Verification items for this drawing (mm, ordinates from the low corner). Round coordinates to 2 decimals unless told otherwise and drop trailing zeros. Write each loop counter-clockwise with the first axis right and the second up, starting at its lowest first coordinate (ties: lowest second). Pieces come first, ordered by that corner, then holes. Notation, with made-up numbers: (-11.5, 66.25) -> (25.5, 66.25) arc R11 ccw to (25.5, 70.25) -> close; hole circle Ø1 at (3, 48.5). An arc over 180 degrees is marked (long way). One line per question, with ' | ' between items.
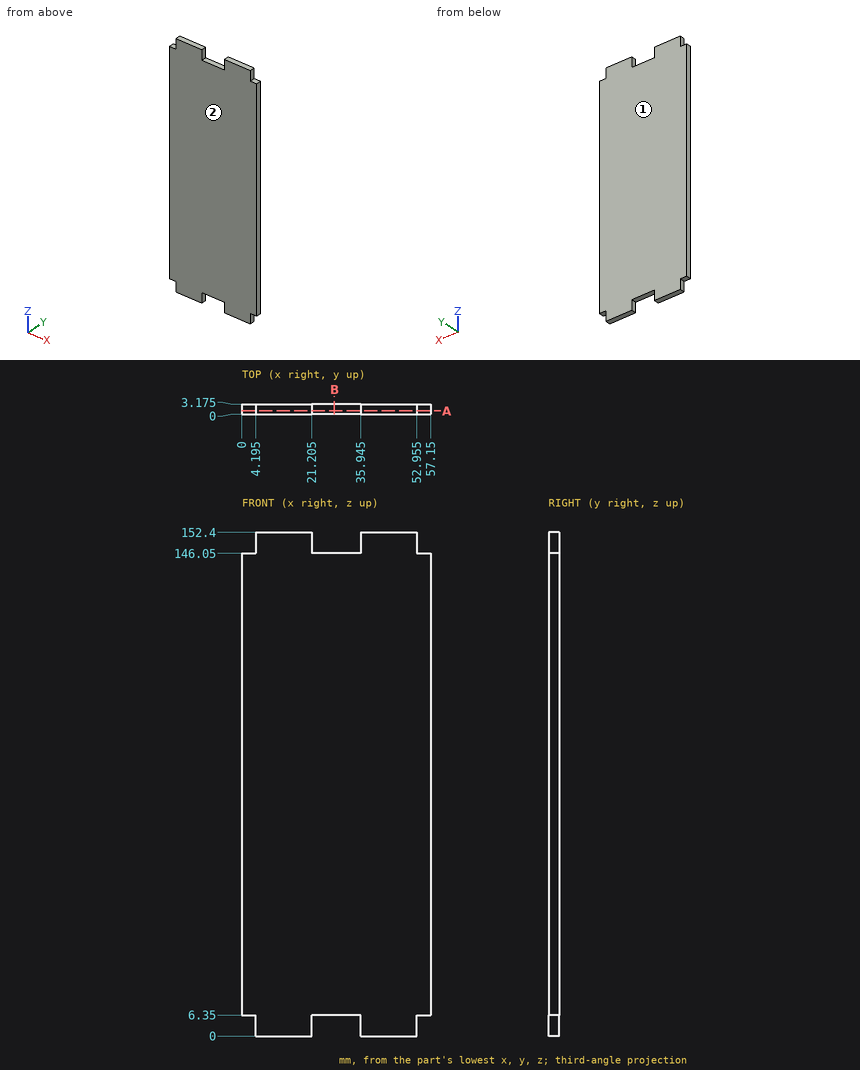
(1) Draft check along Y on the marked faces 1 and 2. Enter one of: +Y half, -Y half, draft (parallel to the pull), parting line (faces both ways), or undercut.
Resolved:
face 1: +Y half | face 2: -Y half
(2) Sectioned sample at B-B on x = 28. Record the cut outline in (y, z) (3 decimals), then the cut area to 3 significant figures.
Resolved:
outline: (0, 6.35) -> (3.175, 6.35) -> (3.175, 146.05) -> (0, 146.05) -> close | area: 444 mm2
(3) Go/stop test with flat-tipped pins: pin 1 (1.6 mm diameter, centred on x = 1.5, y = 2.5, fed in from -Z); pin 2 (1.6 mm diameter, centred on y = 2, z = 2.5, fed in from +X) (3 decimals); pin 3 (1 mm diameter, centred on x = 55.5, y = 1.5, fed in from +Z). Record where each tip stops, or that it passes through.
Resolved:
pin 1: stops at z = 6.35 | pin 2: stops at x = 52.955 | pin 3: stops at z = 146.05
(4) Material ranges on line 1 (X direction, y = 0.2, z = 6) (3 decimals); line 2 (Z direction, x = 33, y = 1), recorded low to high.
Resolved:
line 1: x = 4.195 to 21.205, 35.945 to 52.955 | line 2: z = 6.35 to 146.05
(5) Sectioned sample at A-A on y = 1.1. Record the cut outline in (x, z) (3 decimals), then the cut area to 3 significant figures.
Resolved:
outline: (0, 6.35) -> (4.195, 6.35) -> (4.195, 0) -> (21.205, 0) -> (21.205, 6.35) -> (35.945, 6.35) -> (35.945, 0) -> (52.955, 0) -> (52.955, 6.35) -> (57.15, 6.35) -> (57.15, 146.05) -> (52.955, 146.05) -> (52.955, 152.4) -> (35.945, 152.4) -> (35.945, 146.05) -> (21.205, 146.05) -> (21.205, 152.4) -> (4.195, 152.4) -> (4.195, 146.05) -> (0, 146.05) -> close | area: 8,420 mm2
